```python
from build123d import *

# Parameters (mm, degrees)
F_01_START                                  = -57.2
S01_POLOLU_4755_BRUSHED_MOTOR_CAN_R         = 17.4
F_01_POLOLU_4755_BRUSHED_MOTOR_CAN_DEPTH    = 30.7
F_02_START                                  = -26.5
S02_37D_GEARBOX_BODY_R                      = 18.4
F_02_37D_GEARBOX_BODY_DEPTH                 = 26.5
F_03_START                                  = -3
S03_MANUFACTURER_SIX_M3_FACE_THREADS_R      = 1.52
F_03_MANUFACTURER_SIX_M3_FACE_THREADS_DEPTH = 3.2
S04_FRONT_LOCATING_BOSS_R                   = 6
F_04_FRONT_LOCATING_BOSS_DEPTH              = 6
F_05_START                                  = -72.6
S05_QUADRATURE_ENCODER_REAR_CAP_15_4_R      = 17
F_05_QUADRATURE_ENCODER_REAR_CAP_15_4_DEPTH = 15.4
F_06_START                                  = 1.6
S06_SHAFT_JOURNAL_AT_GEARBOX_OUTPUT_R       = 2.75
F_06_SHAFT_JOURNAL_AT_GEARBOX_OUTPUT_DEPTH  = 4.5


with BuildPart() as part:
    # S01 - Pololu 4755 brushed motor can → 01 - Pololu 4755 brushed motor can (new body)
    with BuildSketch(Plane.XY.offset(F_01_START)):
        with Locations((7, 0)):
            Circle(S01_POLOLU_4755_BRUSHED_MOTOR_CAN_R)
    extrude(amount=F_01_POLOLU_4755_BRUSHED_MOTOR_CAN_DEPTH)

    # S02 - 37D gearbox body → 02 - 37D gearbox body (add)
    with BuildSketch(Plane.XY.offset(F_02_START)):
        with Locations((7, 0)):
            Circle(S02_37D_GEARBOX_BODY_R)
    extrude(amount=F_02_37D_GEARBOX_BODY_DEPTH)

    # S03 - Manufacturer six M3 face threads → 03 - Manufacturer six M3 face threads (cut)
    with BuildSketch(Plane.XY.offset(F_03_START)):
        with Locations((20.423393759, 7.75)):
            Circle(S03_MANUFACTURER_SIX_M3_FACE_THREADS_R)
        with Locations((7, 15.5)):
            Circle(S03_MANUFACTURER_SIX_M3_FACE_THREADS_R)
        with Locations((-6.423393759, 7.75)):
            Circle(S03_MANUFACTURER_SIX_M3_FACE_THREADS_R)
        with Locations((-6.423393759, -7.75)):
            Circle(S03_MANUFACTURER_SIX_M3_FACE_THREADS_R)
        with Locations((7, -15.5)):
            Circle(S03_MANUFACTURER_SIX_M3_FACE_THREADS_R)
        with Locations((20.423393759, -7.75)):
            Circle(S03_MANUFACTURER_SIX_M3_FACE_THREADS_R)
    extrude(amount=F_03_MANUFACTURER_SIX_M3_FACE_THREADS_DEPTH, mode=Mode.SUBTRACT)

    # S04 - Front locating boss → 04 - Front locating boss (add)
    with BuildSketch(Plane.XY):
        Circle(S04_FRONT_LOCATING_BOSS_R)
    extrude(amount=F_04_FRONT_LOCATING_BOSS_DEPTH)

    # S05 - Quadrature encoder rear cap - 15.4 mm → 05 - Quadrature encoder rear cap - 15.4 mm (add)
    with BuildSketch(Plane.XY.offset(F_05_START)):
        with Locations(Location((7, 0, 0), (0, 0, 180))):
            Circle(S05_QUADRATURE_ENCODER_REAR_CAP_15_4_R)
    extrude(amount=F_05_QUADRATURE_ENCODER_REAR_CAP_15_4_DEPTH)

    # S06 - Shaft journal at gearbox output → 06 - Shaft journal at gearbox output (cut)
    with BuildSketch(Plane.XY.offset(F_06_START)):
        Circle(S06_SHAFT_JOURNAL_AT_GEARBOX_OUTPUT_R)
    extrude(amount=F_06_SHAFT_JOURNAL_AT_GEARBOX_OUTPUT_DEPTH, mode=Mode.SUBTRACT)


solid = part.part
```
Here's how the part is built. I have some questions about the finished solid (model axes, mm). A direction names the side the tool comes from. Give positions to 0.01 mm unless a question says otherwise; leave off trailing zeros. Write each loop counter-clockwise with the first axis right and the second up, starting at its lowest first coordinate (ties: lowest second). Pieces come first, ordered by that corner, then holes. Notation, with made-up numbers: M 29,5.5 L 37,5.5 A20 ccw 37,27.5 Z; hole C 30,-35.75 d8. An arc over 180 degrees is marked long. Put each result on its own line as item: value. Start each with the question number.
Item 1: If we section it at C-C, the plane z = -10.5: Write out the boundary of the cut face in (x, y).
Item 2: If we section it at A-A, the plane x = 7: Write out the boundary of the cut face in (y, z).
Item 3: If we section it at B-B, the plane y = 10.5: Write out the boundary of the cut face in (x, z).
Item 4: I need wall thicknesses on L1, parallel to Y at x = 7, z = -1; L2, parallel to Z at x = 10.5, y = -7.5; L3, parallel to X at y = 7, z = -2. Which ranges of each line are inside material? Lowest first, please. Write a range as from..to.
Item 5: Thinking about a two-plate mould opening in X: for faces 4 (the cylindrical face through (15.029, -15.437, -42.065)), 5 (the cylindrical face through (5.88, 16.53, -1.52)), 6 (the flat face through (3, -1, 6)), which applies, +X half, -X half, draft (parallel to the pull), parting line (faces both ways), or undercut?
Item 6: On a 3-axis mill with a long thin cutter (end or side, diameter ignored), from which of +Z, -Z, +X, -X, +Y, -Y can I reach the whole of each face in a straight line? I mean faces 1 (the flat face through (22.4, -7.7, -57.2)), 2 (the cylindrical face through (-4.974, -7.293, -1.521)), 3 (the flat face through (7, 0, -72.6)). Say none if no direction works.
Item 7: Will these pins go through, and if not, where does the flat tip stop? pin 1 (5 mm diameter, centred on y = 5.5, z = -54.5, fed in from +X); pin 2 (10 mm diameter, centred on x = 20.5, z = -49.5, fed in from -Y); pin 3 (3 mm diameter, centred on y = -3.5, z = -33, fed in from +X).
Item 8: If we section it at D-D, the plane x = 0: Write out the boundary of the cut face in (y, z), then the cut area to 3 significant figures.
Values:
1. outline: C 7,0 d36.8
2. outline: M -18.4,-26.5 L -17.4,-26.5 L -17.4,-57.2 L -17,-57.2 L -17,-72.6 L 17,-72.6 L 17,-57.2 L 17.4,-57.2 L 17.4,-26.5 L 18.4,-26.5 L 18.4,0 L 17.02,0 L 17.02,-3 L 13.98,-3 L 13.98,0 L -13.98,0 L -13.98,-3 L -17.02,-3 L -17.02,0 L -18.4,0 Z
3. outline: M -8.11,-26.5 L -6.87,-26.5 L -6.87,-57.2 L -6.37,-57.2 L -6.37,-72.6 L 20.37,-72.6 L 20.37,-57.2 L 20.87,-57.2 L 20.87,-26.5 L 22.11,-26.5 L 22.11,0 L -8.11,0 Z
4. L1: -18.4..-17.02, -13.98..13.98, 17.02..18.4
4. L2: -72.6..0
4. L3: -10.02..-7.75, -5.1..19.1, 21.75..24.02
5. face 4: parting line
5. face 5: undercut
5. face 6: draft
6. face 1: -Z
6. face 2: +Z
6. face 3: -Z, +X, -X, +Y, -Y
7. pin 1: x = 24.14
7. pin 2: y = -15.18
7. pin 3: x = 24.28
8. outline: M -17.02,-26.5 L -15.93,-26.5 L -15.93,-57.2 L -15.49,-57.2 L -15.49,-72.6 L 15.49,-72.6 L 15.49,-57.2 L 15.93,-57.2 L 15.93,-26.5 L 17.02,-26.5 L 17.02,0 L 6,0 L 6,6 L 2.75,6 L 2.75,1.6 L -2.75,1.6 L -2.75,6 L -6,6 L -6,0 L -17.02,0 Z
8. area: 2,400 mm²
